Input: dimensioned drawing with shaded views. Units: mm. Origin: part minimum x, y, z. Round coordinates to 2 decimals unless told otherwise and drop trailing zeros. Write each loop counter-clockwise with the first axis right and the second up, starting at its lowest first coordinate (ties: lowest second). Pieces come first, ordered by that corner, then holes. Notation, with made-up numbers: M -39,-5 L -31,-5 A13 ccw -31,17 Z; hole C 40,55 d7. An arc over 180 degrees is marked long. Answer in a Markdown table with one row per item. Add a question column.
Item 1: Cut plane D-D on z = 10. Return loops of the section in (x, y) (1 decimal).
Item 2: Contact query for flat-ended pins moving along their axis: pin 1 (10 mm diameter, centred on x = 45.34, y = 75.96, fed in from +Z) (3 decimals); pin 2 (5 mm diameter, centred on x = 51, z = 16, fed in from +Y); pin 3 (5 mm diameter, centred on x = 13.5, z = 3.5, fed in from +Y). Output: stop coordinate, or through.
Item 3: Cut plane B-B on y = 75. Return loops of the section in (x, z) (1 decimal), and give its area (3 significant figures).
Item 4: Material intervals for probe 1 along Z at (x, y) = (13, 12) (1 decimal); probe 2 along Y at (x, z) = (36, 5.5) (1 decimal); probe 3 along X at (y, z) = (46.5, 6), sorted ascending.
Item 5: Cut plane A-A on x = 14.5. Return loops of the section in (y, z) (1 decimal), and give its area (3 significant figures).
Item 6: Mould query, pull axis X, two halves, no side actions, for the marked faces 1, 2 and 3. Classes: released by +X, released by -X, zero draft, split by the parting line, or undercut.
Item 7: Cut plane C-C on z = 2. Give the number of separate pieces and of enclosed holes in the cut face, and give its area (3 significant figures).
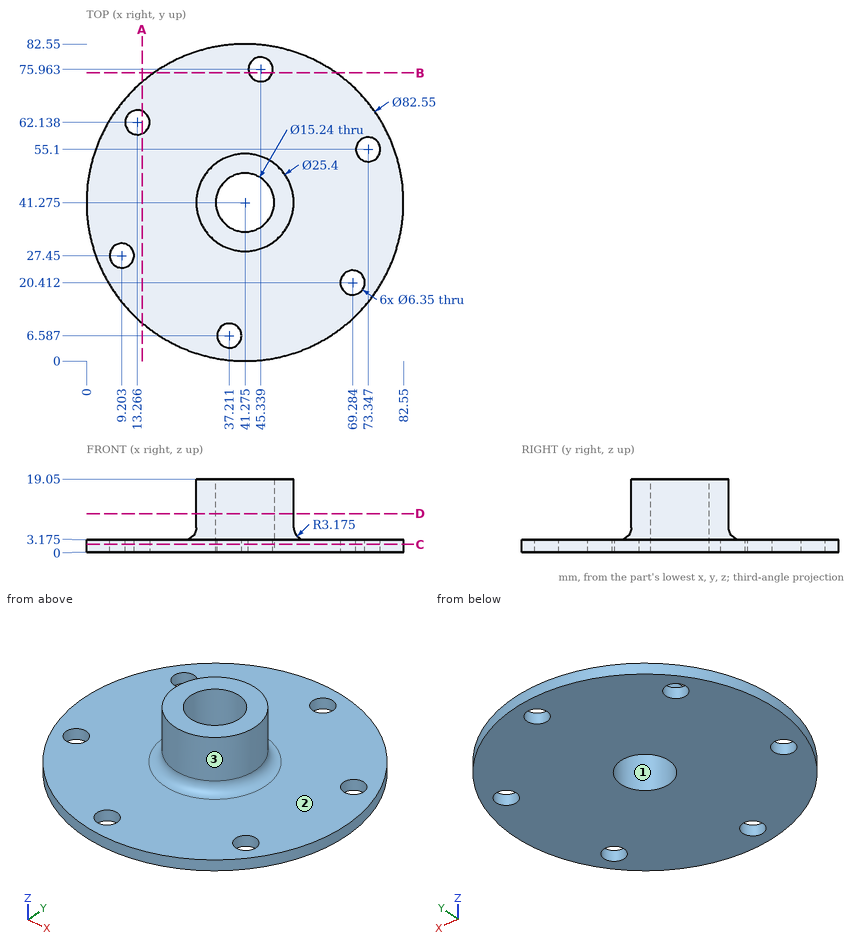
Results below:
| question | item | result |
|---|---|---|
| 1 | outline | C 41.3,41.3 d25.4; hole C 41.3,41.3 d15.2 |
| 2 | pin 1 | z = 3.175 |
| 2 | pin 2 | y = 51.72 |
| 2 | pin 3 | y = 73.89 |
| 3 | outline | M 17.5,0 L 42.3,0 L 42.3,3.2 L 17.5,3.2 Z; M 48.4,0 L 65.1,0 L 65.1,3.2 L 48.4,3.2 Z |
| 3 | area | 132 mm2 |
| 4 | probe 1 | 0 to 3.2 |
| 4 | probe 2 | 29.6 to 35.8, 46.8 to 53 |
| 4 | probe 3 | 29.68 to 35.73, 46.82 to 52.87 |
| 5 | outline | M 9.9,0 L 59.2,0 L 59.2,3.2 L 9.9,3.2 Z; M 65.1,0 L 72.7,0 L 72.7,3.2 L 65.1,3.2 Z |
| 5 | area | 181 mm2 |
| 6 | face 1 | undercut |
| 6 | face 2 | zero draft |
| 6 | face 3 | split by the parting line |
| 7 | separate pieces | 1 |
| 7 | enclosed holes | 7 |
| 7 | area | 4,980 mm2 |
